Geometry: final body of the model. Coordinates: model frame, mm. A direction names the side the tool comes from. Give positions to 0.01 mm unless a question says otherwise; leave off trailing zeros. Write each loop counter-clockwise with the first axis right and the second up, starting at its lowest first coordinate (ties: lowest second). Pieces come first, ordered by that corner, then holes. Notation, with made-up numbers: M 37.5,13.5 L 77.5,13.5 A7 cw 77.5,26.5 Z; hole C 40.25,72.5 d7. An arc over 180 degrees is marked long. Answer as a JSON object with one key per item and string values.
from build123d import *

# Parameters (mm, degrees)
SKETCH1_R                = 30.1625
SKETCH1_R_2              = 26.9875
BOSS_EXTRUDE1_DEPTH      = 1.5875
BOSS_EXTRUDE2_START      = -1.5875
SKETCH2_R                = 2.4892
BOSS_EXTRUDE2_DEPTH      = 1.5875
CIRPATTERN1_COUNT        = 6
BOSS_EXTRUDE3_START      = -1.5875
BOSS_EXTRUDE3_DEPTH      = 1.5875
FILLET1_R                = 2.286
FILLET2_R                = 1.524
FILLET3_R                = 0.635
CIRPATTERN2_COUNT        = 8
FILLET1_OF_CIRPATTERN2_R = 2.286
FILLET2_OF_CIRPATTERN2_R = 1.524
FILLET3_OF_CIRPATTERN2_R = 0.635


with BuildPart() as part:
    # Sketch1 → Boss-Extrude1 (new body)
    with BuildSketch(Plane(origin=(0, 0, 0), x_dir=(1, 0, 0), z_dir=(0, 1, 0))):
        with Locations(Location((0, 0, 0), (0, 0, 270))):
            Circle(SKETCH1_R)
        with Locations(Location((0, 0, 0), (0, 0, 270))):
            Circle(SKETCH1_R_2, mode=Mode.SUBTRACT)
    extrude(amount=BOSS_EXTRUDE1_DEPTH)

    # Sketch2 → Boss-Extrude2 (add)
    with BuildSketch(Plane(origin=(0, 1.5875, 0), x_dir=(1, 0, 0), z_dir=(0, 1, 0)).offset(BOSS_EXTRUDE2_START)):
        with BuildLine():
            ThreePointArc((-9.237332215, 25.35738255), (-6.184469909, 24.956114415), (-4.7625, 22.225))
            ThreePointArc((-4.7625, 22.225), (0, 17.4625), (4.7625, 22.225))
            ThreePointArc((4.7625, 22.225), (6.184469909, 24.956114415), (9.237332215, 25.35738255))
            ThreePointArc((9.237332215, 25.35738255), (0, 26.9875), (-9.237332215, 25.35738255))
        make_face()
        with Locations(Location((0, 22.225, 0), (0, 0, 270))):
            Circle(SKETCH2_R, mode=Mode.SUBTRACT)
    boss_extrude2 = extrude(amount=BOSS_EXTRUDE2_DEPTH)

    # CirPattern1: Boss-Extrude2 ×6 about axis
    cirpattern1_axis = Axis((0, 0, 0), (0, 1, 0))
    for i in range(1, CIRPATTERN1_COUNT):
        add(boss_extrude2.rotate(cirpattern1_axis, i * 360 / CIRPATTERN1_COUNT))

    # Sketch3 → Boss-Extrude3 (add)
    with BuildSketch(Plane(origin=(0, 1.5875, 0), x_dir=(1, 0, 0), z_dir=(0, 1, 0)).offset(BOSS_EXTRUDE3_START)):
        with BuildLine():
            Line((4.517012817, 32.486934384), (0, 30.1625))
            ThreePointArc((0, 30.1625), (1.589709482, 30.120578182), (3.175, 29.994929259))
            ThreePointArc((3.175, 29.994929259), (3.206558857, 30.078714629), (3.175, 30.1625))
            Line((3.175, 30.1625), (4.517012817, 32.486934384))
        make_face()
        with BuildLine():
            Line((-4.517012817, 32.486934384), (-3.175, 30.1625))
            ThreePointArc((-3.175, 30.1625), (-3.206558857, 30.078714629), (-3.175, 29.994929259))
            ThreePointArc((-3.175, 29.994929259), (-1.589709482, 30.120578182), (0, 30.1625))
            Line((0, 30.1625), (-4.517012817, 32.486934384))
        make_face()
    boss_extrude3 = extrude(amount=BOSS_EXTRUDE3_DEPTH)

    # Fillet1
    fillet1_edges = [part.edges().sort_by_distance(p)[0] for p in [
        (0, 0.79375, -30.1625),
    ]]
    fillet(fillet1_edges, radius=FILLET1_R)

    # Fillet2
    # the kernel refuses this fillet: 1.524 mm, written as the material it adds along each edge
    with BuildSketch(Plane(origin=(3.175, 0, -29.994929259), x_dir=(0, 0, -1), z_dir=(0, 1, 0))) as fillet2_piece_1:
        with BuildLine():
            CenterArc((1.435454488, -0.845604401), FILLET2_R, 146.299028695, 26.411231524)
            Line((-0.076227295, -0.652228639), (-0.106460931, -0.648361123))
            ThreePointArc((-0.106460931, -0.648361123), (-0.06661258, -0.322783591), (-0.030310665, 0.003208421))
            Line((-0.030310665, 0.003208421), (0.020108489, 0.022905874))
            ThreePointArc((0.020108489, 0.022905874), (0.083785371, -0.001078857), (0.142213066, 0.016912088))
            Line((0.142213066, 0.016912088), (0.167570741, 0))
        make_face()
    extrude(amount=1.5875)
    with BuildSketch(Plane(origin=(-3.175, 0, -29.994929259), x_dir=(-0.9932396393904435, 0, 0.11608194839656201), z_dir=(0, 1, 0))) as fillet2_piece_2:
        with BuildLine():
            CenterArc((0.673257457, -1.523909705), FILLET2_R, 90.623705681, 26.411231524)
            Line((-0.019451938, -0.166437902), (-0.033306126, -0.139288466))
            ThreePointArc((-0.033306126, -0.139288466), (-0.008654405, -0.083344187), (-0.025085255, -0.01731359))
            Line((-0.025085255, -0.01731359), (0.00033179, 0.030478194))
            ThreePointArc((0.00033179, 0.030478194), (0.328333975, 0.028692907), (0.656336161, 0.030478194))
            Line((0.656336161, 0.030478194), (0.656667951, 0))
        make_face()
    extrude(amount=1.5875)

    # Fillet3
    fillet3_edges = [part.edges().sort_by_distance(p)[0] for p in [
        (-3.175, 0.79375, -30.1625),
        (3.175, 0.79375, -30.1625),
    ]]
    fillet(fillet3_edges, radius=FILLET3_R)

    # CirPattern2: Boss-Extrude3 ×8 about axis
    cirpattern2_axis = Axis((0, 0, 0), (0, 1, 0))
    for i in range(1, CIRPATTERN2_COUNT):
        add(boss_extrude3.rotate(cirpattern2_axis, i * 360 / CIRPATTERN2_COUNT))

    # Fillet1 of CirPattern2
    fillet1_of_cirpattern2_edges = [part.edges().sort_by_distance(p)[0] for p in [
        (-21.328108288, 0.79375, -21.328108288),
        (-30.1625, 0.79375, 0),
        (-21.328108288, 0.79375, 21.328108288),
        (0, 0.79375, 30.1625),
        (21.328108288, 0.79375, 21.328108288),
        (30.1625, 0.79375, 0),
        (21.328108288, 0.79375, -21.328108288),
    ]]
    fillet(fillet1_of_cirpattern2_edges, radius=FILLET1_OF_CIRPATTERN2_R)

    # Fillet2 of CirPattern2
    # the kernel refuses this fillet: 1.524 mm, written as the material it adds along each edge
    with BuildSketch(Plane(origin=(-18.96455385, 0, -23.45468191), x_dir=(0.7844088172408243, 0, -0.6202441514717015), z_dir=(0, 1, 0)), Plane(origin=(-29.994929259, 0, -3.175), x_dir=(0.11608194839659203, 0, -0.9932396393904398), z_dir=(0, 1, 0)), Plane(origin=(-23.45468191, 0, 18.96455385), x_dir=(-0.620244151471689, 0, -0.7844088172408342), z_dir=(0, 1, 0))) as fillet2_of_cirpattern2_piece_1:
        with BuildLine():
            CenterArc((0.673257457, 1.523909705), FILLET2_OF_CIRPATTERN2_R, 242.965062795, 26.411231524)
            Line((-0.019451938, 0.166437902), (-0.033306126, 0.139288466))
            ThreePointArc((-0.033306126, 0.139288466), (-0.008654405, 0.083344187), (-0.025085255, 0.01731359))
            Line((-0.025085255, 0.01731359), (0.00033179, -0.030478194))
            ThreePointArc((0.00033179, -0.030478194), (0.328333975, -0.028692907), (0.656336161, -0.030478194))
            Line((0.656336161, -0.030478194), (0.656667951, 0))
        make_face()
    extrude(amount=1.5875)
    with BuildSketch(Plane(origin=(-23.45468191, 0, -18.96455385), x_dir=(-0.7071067811865793, 0, -0.7071067811865157), z_dir=(0, 1, 0)), Plane(origin=(-29.994929259, 0, 3.175), x_dir=(-1, 0, 0), z_dir=(0, 1, 0)), Plane(origin=(18.96455385, 0, -23.45468191), x_dir=(0.7071067811865369, 0, -0.7071067811865581), z_dir=(0, 1, 0))) as fillet2_of_cirpattern2_piece_2:
        with BuildLine():
            CenterArc((1.435454488, 0.845604401), FILLET2_OF_CIRPATTERN2_R, 187.289739781, 26.411231524)
            Line((-0.076227295, 0.652228639), (-0.106460931, 0.648361123))
            ThreePointArc((-0.106460931, 0.648361123), (-0.06661258, 0.322783591), (-0.030310665, -0.003208421))
            Line((-0.030310665, -0.003208421), (0.020108489, -0.022905874))
            ThreePointArc((0.020108489, -0.022905874), (0.083785371, 0.001078857), (0.142213066, -0.016912088))
            Line((0.142213066, -0.016912088), (0.167570741, 0))
        make_face()
    extrude(amount=1.5875)
    with BuildSketch(Plane(origin=(-18.96455385, 0, 23.45468191), x_dir=(0.784408817240829, 0, 0.6202441514716955), z_dir=(0, 1, 0)), Plane(origin=(3.175, 0, 29.994929259), x_dir=(0.9932396393904444, 0, -0.11608194839655256), z_dir=(0, 1, 0)), Plane(origin=(23.45468191, 0, 18.96455385), x_dir=(0.6202441514717251, 0, -0.7844088172408058), z_dir=(0, 1, 0)), Plane(origin=(29.994929259, 0, -3.175), x_dir=(-0.1160819483965305, 0, -0.9932396393904471), z_dir=(0, 1, 0))) as fillet2_of_cirpattern2_piece_3:
        with BuildLine():
            CenterArc((0.673257457, -1.523909705), FILLET2_OF_CIRPATTERN2_R, 90.623705681, 26.411231524)
            Line((-0.019451938, -0.166437902), (-0.033306126, -0.139288466))
            ThreePointArc((-0.033306126, -0.139288466), (-0.008654405, -0.083344187), (-0.025085255, -0.01731359))
            Line((-0.025085255, -0.01731359), (0.00033179, 0.030478194))
            ThreePointArc((0.00033179, 0.030478194), (0.328333975, 0.028692907), (0.656336161, 0.030478194))
            Line((0.656336161, 0.030478194), (0.656667951, 0))
        make_face()
    extrude(amount=1.5875)
    with BuildSketch(Plane(origin=(-3.175, 0, 29.994929259), x_dir=(0, 0, 1), z_dir=(0, 1, 0)), Plane(origin=(18.96455385, 0, 23.45468191), x_dir=(0.7071067811865263, 0, 0.7071067811865687), z_dir=(0, 1, 0)), Plane(origin=(29.994929259, 0, 3.175), x_dir=(1, 0, 0), z_dir=(0, 1, 0)), Plane(origin=(23.45468191, 0, -18.96455385), x_dir=(0.7071067811865581, 0, -0.7071067811865369), z_dir=(0, 1, 0))) as fillet2_of_cirpattern2_piece_4:
        with BuildLine():
            CenterArc((1.435454488, -0.845604401), FILLET2_OF_CIRPATTERN2_R, 146.299028695, 26.411231524)
            Line((-0.076227295, -0.652228639), (-0.106460931, -0.648361123))
            ThreePointArc((-0.106460931, -0.648361123), (-0.06661258, -0.322783591), (-0.030310665, 0.003208421))
            Line((-0.030310665, 0.003208421), (0.020108489, 0.022905874))
            ThreePointArc((0.020108489, 0.022905874), (0.083785371, -0.001078857), (0.142213066, 0.016912088))
            Line((0.142213066, 0.016912088), (0.167570741, 0))
        make_face()
    extrude(amount=1.5875)

    # Fillet3 of CirPattern2
    fillet3_of_cirpattern2_edges = [part.edges().sort_by_distance(p)[0] for p in [
        (-23.573172318, 0.79375, -19.083044257),
        (-19.083044257, 0.79375, -23.573172318),
        (-30.1625, 0.79375, 3.175),
        (-30.1625, 0.79375, -3.175),
        (-19.083044257, 0.79375, 23.573172318),
        (-23.573172318, 0.79375, 19.083044257),
        (3.175, 0.79375, 30.1625),
        (-3.175, 0.79375, 30.1625),
        (23.573172318, 0.79375, 19.083044257),
        (19.083044257, 0.79375, 23.573172318),
        (30.1625, 0.79375, -3.175),
        (30.1625, 0.79375, 3.175),
        (19.083044257, 0.79375, -23.573172318),
        (23.573172318, 0.79375, -19.083044257),
    ]]
    fillet(fillet3_of_cirpattern2_edges, radius=FILLET3_OF_CIRPATTERN2_R)


solid = part.part
1) Line query: line 1 (X direction, y = 0.25, z = -10.5); line 2 (X direction, y = 0.95, z = -23); line 3 (Z direction, x = 16, y = 1.4). Output: solid intervals per line, ascending. Write a range as from..to.
Geometry check:
{"line 1": "x = -28.28..-21.66, -16.83..-14.52, 14.52..16.83, 21.66..28.28", "line 2": "x = -20.79..-14.12, -4.85..-2.37, 2.37..4.85, 14.12..20.79", "line 3": "z = -25.57..-21.73, -14.6..-7.63, 7.63..14.6, 21.73..25.57"}
2) Contact query for a flat-ended pin moving along its axis: P1, Ø3, axis at x = 0, z = 22.225, coming from the -Y side. Output: stop coordinate, or through.
Geometry check:
{"P1": "passes through"}
3) Cut plane C-C on x = -13. Return loops of the section in (y, z), and give its area (3 significant figures).
Geometry check:
{"outline": "M 0,-27.22 L 1.59,-27.22 L 1.59,-23.65 L 0,-23.65 Z; M 0,23.65 L 1.59,23.65 L 1.59,27.22 L 0,27.22 Z", "area": "11.3 mm2"}
4) Cut plane D-D on y = 0.55. Give the number of separate pieces and of enclosed holes in the cut face, and give its area (3 significant figures).
Geometry check:
{"separate pieces": "1", "enclosed holes": "7", "area": "1,050 mm2"}
5) Cut plane B-B on z = -2.5. Return loops of the section in (x, y).
Geometry check:
{"outline": "M -31.45,0 L -26.87,0 L -26.87,1.59 L -31.45,1.59 Z; M 26.87,0 L 31.45,0 L 31.45,1.59 L 26.87,1.59 Z"}
6) Pull-direction query (X, two-part tool) for faces 1 (the flat face through (4.048, 0.783, 31.674)), 2 (the flat face through (-20.365, 0.783, -24.333)), 3 (the flat face through (2.81, 0.78, -31.61)); classes: pulls with the +X half, pulls with the -X half, needs draft (parallel to the pull), parting line crosses it, or undercut.
Geometry check:
{"face 1": "pulls with the +X half", "face 2": "pulls with the -X half", "face 3": "undercut"}
7) Cut plane A-A on x = 0. Return loops of the section in (y, z).
Geometry check:
{"outline": "M 0,-30.45 L 1.59,-30.45 L 1.59,-24.71 L 0,-24.71 Z; M 0,-19.74 L 1.59,-19.74 L 1.59,-17.46 L 0,-17.46 Z; M 0,17.46 L 1.59,17.46 L 1.59,19.74 L 0,19.74 Z; M 0,24.71 L 1.59,24.71 L 1.59,30.45 L 0,30.45 Z"}
8) Set-up query: faces 4 (the flat face through (19.528, 0.783, 25.234)), 5 (the cylindrical face through (18.524, 0.783, -17.879)), 6 (the flat face through (-25.234, 0.783, 19.528)). Return all of +Z, -Z, +X, -X, +Y, -Y with unobstructed straight access to the full face (end or side cutting, diameter ignored); none if empty.
Geometry check:
{"face 4": "+Z, +Y, -Y", "face 5": "+Y, -Y", "face 6": "-X, +Y, -Y"}
